Verification items for the finished model (mm, model axes). Face numbers are marked on the shaded views. A direction names the side the tool comes from. Give positions to 0.01 mm unless a question says otherwise; leave off trailing zeros. Loops run counter-clockwise (first coordinate to the right, second up) from the corner with the lowest first, then second, coordinate; pieces in that order, holes last. Notation, with made-up numbers: (68, 33) - (86, 33) arc R17 cw to (86, 37) - close; hole circle Ø5 at (6.5, 9). An arc over 180 degrees is marked (long way). One line per question, with ' | ' between items. Start each with the question number.
1. Section check C-C, the plane x = -468.5. Enter the section's corners in (y, z).
2. Section check B-B, the plane z = -83. Enter the section's corners in (x, y), then the cut area to 3 significant figures.
3. Thickness scan on line 1 along Y through (x, z) = (261, 285); line 2 along X through (y, z) = (-228.5, 119); line 3 along Z through (x, y) = (249, -416). Record the ranges inside material, lowest first. Write a range as from..to.
4. Depth check by flat-ended pin: pin 1 Ø1.5 at (x, z) = (-188, 134.5) entering from -Y; pin 2 Ø6 at (x, y) = (-409, -335.5) entering from -Z; pin 3 Ø1 at (y, z) = (-182, -392) entering from +X. Enter the tip coordinate at first touch or a pass-through.
5. Section check A-A, the plane y = 45. Enter the section's corners in (x, z).
6. Tool access check on the marked faces 1, 2 and 3. Record the directions out of +Z, -Z, +X, -X, +Y, -Y that give a thin tool (end or side, any length) a straight path to the whole face; none if there is none.
7. Section check D-D, the plane y = -318. Enter the section's corners in (x, z).
from build123d import *

# Parameters (mm, degrees)
F0_W     = 1500
F0_H     = 1000
F1_DEPTH = 25
F3_DEPTH = 100
F4_W     = 1500
F4_H     = 5
F5_DEPTH = 500
F7_DEPTH = 500


with BuildPart() as f1:
    # F0 (on Front) → F1 (new body, symmetric)
    with BuildSketch(Plane.XZ):
        Rectangle(F0_W, F0_H)
    extrude(amount=F1_DEPTH, both=True)

    # F2 (on face) → F3 (join)
    with BuildSketch(Plane(origin=(0, 25, 0), x_dir=(-1, 0, 0), z_dir=(0, 1, 0))):
        Polygon((700, -500), (750, -500), (750, -450), (745, -450), (745, -495), (700, -495), align=None)
        Polygon((-750, -500), (-700, -500), (-700, -495), (-745, -495), (-745, -450), (-750, -450), align=None)
        Polygon((-700, 495), (-700, 500), (-750, 500), (-750, 450), (-745, 450), (-745, 495), align=None)
        Polygon((745, 450), (750, 450), (750, 500), (700, 500), (700, 495), (745, 495), align=None)
    extrude(amount=F3_DEPTH)

    # F4 (on face) → F5 (join)
    with BuildSketch(Plane.XZ.offset(25)):
        with Locations((0, 497.5)):
            Rectangle(F4_W, F4_H)
    extrude(amount=F5_DEPTH)

    # F6 (on face) → F7 (join)
    with BuildSketch(Plane.XZ.offset(25)):
        Polygon((-5, -500), (0, -500), (5, -500), (5, 495), (0, 495), (-5, 495), align=None)
    extrude(amount=F7_DEPTH)


solid = f1.part
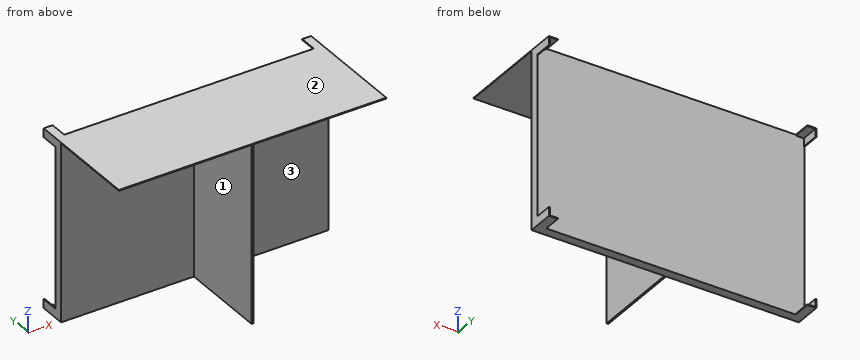
Results list:
1) outline: (-525, 495) - (-25, 495) - (-25, -500) - (25, -500) - (25, 500) - (-525, 500) - close
2) outline: (-750, -25) - (-5, -25) - (-5, -525) - (5, -525) - (5, -25) - (750, -25) - (750, 25) - (-750, 25) - close | area: 80,000 mm²
3) line 1: -25..25 | line 2: -5..5 | line 3: 495..500
4) pin 1: y = -25 | pin 2: z = 495 | pin 3: x = 5
5) outline: (-750, -500) - (-700, -500) - (-700, -495) - (-745, -495) - (-745, -450) - (-750, -450) - close; (-750, 450) - (-745, 450) - (-745, 495) - (-700, 495) - (-700, 500) - (-750, 500) - close; (700, -500) - (750, -500) - (750, -450) - (745, -450) - (745, -495) - (700, -495) - close; (700, 495) - (745, 495) - (745, 450) - (750, 450) - (750, 500) - (700, 500) - close
6) face 1: -Z, -X, -Y | face 2: +Z, +X, -X, +Y, -Y | face 3: -Z, +X, -Y
7) outline: (-750, 495) - (-5, 495) - (-5, -500) - (5, -500) - (5, 495) - (750, 495) - (750, 500) - (-750, 500) - close
